The model under review builds one solid part; all positions refer to its coordinate system, in mm. Face numbers are marked on the shaded views. Round coordinates to 2 decimals unless told otherwise and drop trailing zeros. Write each loop counter-clockwise with the first axis right and the second up, starting at its lowest first coordinate (ties: lowest second). Pieces come first, ordered by that corner, then holes. Notation, with made-up numbers: (32, -21.75) -> (61, -21.75) arc R34 ccw to (61, 8.25) -> close; hole circle Ø5 at (63.5, -39.75). An arc over 180 degrees is marked (long way). Answer in a Markdown table with one row per item. Add a question column.
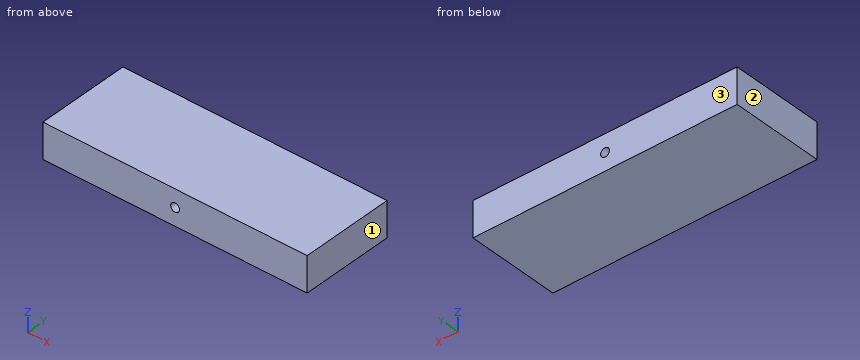
```python
from build123d import *

# Parameters (mm, degrees)
SKETCH_1_W               = 150
SKETCH_1_H               = 53
EXTRUDE_1_DEPTH          = 10
CUT_EXTRUDE_1_DEPTH      = 81.170131595
CUT_EXTRUDE_1_DEPTH_BACK = 81.170131595
SKETCH_2_R               = 2.5


with BuildPart() as part:
    # Эскиз1 → Бобышка-Вытянуть1 (new, symmetric)
    with BuildSketch(Plane.XY):
        Rectangle(SKETCH_1_W, SKETCH_1_H)
    extrude(amount=EXTRUDE_1_DEPTH, both=True)

    # Эскиз2 → Вырез-Вытянуть1 (cut, two sides: drawn at the far end of the back side and taken through both)
    with BuildSketch(Plane(origin=(0, 0, 0), x_dir=(1, 0, 0), z_dir=(0, 1, 0)).offset(-CUT_EXTRUDE_1_DEPTH_BACK)):
        with Locations(Location((0, 0, 0), (0, 0, 270))):
            Circle(SKETCH_2_R)
    extrude(amount=CUT_EXTRUDE_1_DEPTH + CUT_EXTRUDE_1_DEPTH_BACK, mode=Mode.SUBTRACT)


solid = part.part
```
1. Add section B-B on z = 0. Write out the cut boundary in (x, y).
2. Add section A-A on x = 0. Write out the cut boundary in (y, z), plus the area to 3 significant figures.
3. Mouldability with a two-part tool opening along X and no side actions: class the marked faces 1, 2 and 3 as pulls with the +X half, pulls with the -X half, needs draft (parallel to the pull), parting line crosses it, or undercut.
4. For L1, parallel to X at y = -24, z = 0; L2, parallel to Z at x = 0, y = -10.5; L3, parallel to X at y = 3, z = -2, list the stretches that pass through material, from the lowest coordinate up.
Filled in:
| question | item | result |
|---|---|---|
| 1 | outline | (-75, -26.5) -> (-2.5, -26.5) -> (-2.5, 26.5) -> (-75, 26.5) -> close; (2.5, -26.5) -> (75, -26.5) -> (75, 26.5) -> (2.5, 26.5) -> close |
| 2 | outline | (-26.5, -10) -> (26.5, -10) -> (26.5, -2.5) -> (-26.5, -2.5) -> close; (-26.5, 2.5) -> (26.5, 2.5) -> (26.5, 10) -> (-26.5, 10) -> close |
| 2 | area | 795 mm² |
| 3 | face 1 | pulls with the +X half |
| 3 | face 2 | pulls with the -X half |
| 3 | face 3 | needs draft |
| 4 | L1 | -75 to -2.5, 2.5 to 75 |
| 4 | L2 | -10 to -2.5, 2.5 to 10 |
| 4 | L3 | -75 to -1.5, 1.5 to 75 |
